from build123d import *

# Parameters (mm, degrees)
SKETCH1_W                  = 60
SKETCH1_H                  = 60
BOSS_EXTRUDE1_DEPTH        = 80
CUT_EXTRUDE2_START         = -16
SKETCH3_R                  = 11
CUT_EXTRUDE2_DEPTH         = 107.553851381
SKETCH4_OUTSIDE_W          = 105.324
SKETCH4_OUTSIDE_H          = 85.324
SKETCH4_OUTSIDE_W_2        = 47.6
SKETCH4_OUTSIDE_H_2        = 47.6
CUT_EXTRUDE5_DEPTH         = 13
M4_TAPPED_HOLE2_AT_2_COUNT = 2
M4_TAPPED_HOLE2_AT_2_PITCH = 20.8
CIRPATTERN2_COUNT          = 4
CIRPATTERN4_COUNT          = 4
SKETCH21_R                 = 8
CUT_EXTRUDE6_DEPTH         = 77.785415282
SKETCH24_W                 = 10
SKETCH24_H                 = 60
CUT_EXTRUDE7_DEPTH         = 53
SKETCH25_W                 = 60
SKETCH25_H                 = 60
BOSS_EXTRUDE2_DEPTH        = 11
FILLET1_R                  = 2


with BuildPart() as part:
    # Sketch1 → Boss-Extrude1 (new body)
    with BuildSketch(Plane.XY):
        Rectangle(SKETCH1_W, SKETCH1_H)
    extrude(amount=BOSS_EXTRUDE1_DEPTH)

    # Sketch3 → Cut-Extrude2 (cut)
    with BuildSketch(Plane(origin=(0, 0, 0), x_dir=(-1, 0, 0), z_dir=(0, 0, -1)).offset(CUT_EXTRUDE2_START)):
        with Locations(Location((-12, 0, 0), (0, 0, 180))):
            Circle(SKETCH3_R)
    cut_extrude2 = extrude(amount=CUT_EXTRUDE2_DEPTH, mode=Mode.SUBTRACT)

    # Sketch4 outside → Cut-Extrude5 (cut)
    with BuildSketch(Plane.ZY.offset(30)):
        with Locations((40, 0)):
            Rectangle(SKETCH4_OUTSIDE_W, SKETCH4_OUTSIDE_H)
        with Locations((40, 0)):
            Rectangle(SKETCH4_OUTSIDE_W_2, SKETCH4_OUTSIDE_H_2, mode=Mode.SUBTRACT)
    extrude(amount=-CUT_EXTRUDE5_DEPTH, mode=Mode.SUBTRACT)

    # Sketch19 → M4 Tapped Hole2 (revolve, cut)
    with BuildSketch(Plane(origin=(-24, -23.8, 29.6), x_dir=(0, 0, -1), z_dir=(1, 0, 0))):
        Polygon((0, 0), (0, 12.491420021), (1.65, 11.5), (1.65, 0), align=None)
    m4_tapped_hole2 = revolve(axis=Axis((-24, -30.15, 29.6), (0, 1, 0)), mode=Mode.SUBTRACT)

    # M4 Tapped Hole2 at 2: M4 Tapped Hole2 ×2
    with Locations(*[(0, 0, i * M4_TAPPED_HOLE2_AT_2_PITCH) for i in range(1, M4_TAPPED_HOLE2_AT_2_COUNT)]):
        add(m4_tapped_hole2, mode=Mode.SUBTRACT)

    # CirPattern2: M4 Tapped Hole2 ×4 about axis
    cirpattern2_axis = Axis((-30, 0, 40), (1, 0, 0))
    for i in range(1, CIRPATTERN2_COUNT):
        add(m4_tapped_hole2.rotate(cirpattern2_axis, i * 360 / CIRPATTERN2_COUNT), mode=Mode.SUBTRACT)

    # CirPattern2 copy 1 sketch → CirPattern2 copy 1 (revolve, cut)
    with BuildSketch(Plane(origin=(-24, -10.4, 16.2), x_dir=(0, 1, 0), z_dir=(1, 0, 0))):
        Polygon((0, 0), (0, 12.491420021), (1.65, 11.5), (1.65, 0), align=None)
    revolve(axis=Axis((-24, -10.4, 9.85), (0, 0, 1)), mode=Mode.SUBTRACT)

    # CirPattern2 copy 2 sketch → CirPattern2 copy 2 (revolve, cut)
    with BuildSketch(Plane(origin=(-24, 23.8, 29.6), x_dir=(0, 0, 1), z_dir=(1, 0, 0))):
        Polygon((0, 0), (0, 12.491420021), (1.65, 11.5), (1.65, 0), align=None)
    revolve(axis=Axis((-24, 30.15, 29.6), (0, -1, 0)), mode=Mode.SUBTRACT)

    # CirPattern2 copy 3 sketch → CirPattern2 copy 3 (revolve, cut)
    with BuildSketch(Plane(origin=(-24, 10.4, 63.8), x_dir=(0, -1, 0), z_dir=(1, 0, 0))):
        Polygon((0, 0), (0, 12.491420021), (1.65, 11.5), (1.65, 0), align=None)
    revolve(axis=Axis((-24, 10.4, 70.15), (0, 0, -1)), mode=Mode.SUBTRACT)

    # Mirror2: Cut-Extrude2 across plane
    add(cut_extrude2.mirror(Plane(origin=(0, 0, 40), x_dir=(1, 0, 0), z_dir=(0, 0, -1))), mode=Mode.SUBTRACT)

    # Sketch23 → M3 Tapped Hole1 (revolve, cut)
    with BuildSketch(Plane.YZ.offset(26.073090354)):
        Polygon((0, 0), (0, 25.751075774), (1.25, 25), (1.25, 0), align=None)
    m3_tapped_hole1 = revolve(axis=Axis((26.073090354, 0, -6.35), (0, 0, 1)), mode=Mode.SUBTRACT)

    # CirPattern4: M3 Tapped Hole1 ×4 about axis
    cirpattern4_axis = Axis((12, 0, 0), (0, 0, 1))
    for i in range(1, CIRPATTERN4_COUNT):
        add(m3_tapped_hole1.rotate(cirpattern4_axis, i * 360 / CIRPATTERN4_COUNT), mode=Mode.SUBTRACT)

    # Mirror3: M3 Tapped Hole1 across plane
    add(m3_tapped_hole1.mirror(Plane(origin=(0, 0, 40), x_dir=(1, 0, 0), z_dir=(0, 0, -1))), mode=Mode.SUBTRACT)

    # Mirror3 copy 1 sketch → Mirror3 copy 1 (revolve, cut)
    with BuildSketch(Plane(origin=(12, 14.073090354, 80), x_dir=(-1, 0, 0), z_dir=(0, 1, 0))):
        Polygon((0, 0), (0, -25.751075774), (1.25, -25), (1.25, 0), align=None)
    revolve(axis=Axis((12, 14.073090354, 86.35), (0, 0, 1)), mode=Mode.SUBTRACT)

    # Mirror3 copy 2 sketch → Mirror3 copy 2 (revolve, cut)
    with BuildSketch(Plane(origin=(-2.073090354, 0, 80), x_dir=(0, -1, 0), z_dir=(-1, 0, 0))):
        Polygon((0, 0), (0, -25.751075774), (1.25, -25), (1.25, 0), align=None)
    revolve(axis=Axis((-2.073090354, 0, 86.35), (0, 0, 1)), mode=Mode.SUBTRACT)

    # Mirror3 copy 3 sketch → Mirror3 copy 3 (revolve, cut)
    with BuildSketch(Plane(origin=(12, -14.073090354, 80), x_dir=(1, 0, 0), z_dir=(0, -1, 0))):
        Polygon((0, 0), (0, -25.751075774), (1.25, -25), (1.25, 0), align=None)
    revolve(axis=Axis((12, -14.073090354, 86.35), (0, 0, 1)), mode=Mode.SUBTRACT)

    # Sketch21 → Cut-Extrude6 (cut, through all)
    with BuildSketch(Plane(origin=(0, 0, 16), x_dir=(-1, 0, 0), z_dir=(0, 0, -1))):
        with Locations((-12, 0)):
            Circle(SKETCH21_R)
    extrude(amount=-CUT_EXTRUDE6_DEPTH, mode=Mode.SUBTRACT)

    # Sketch24 → Cut-Extrude7 (cut)
    with BuildSketch(Plane(origin=(30, 0, 0), x_dir=(0, 0, -1), z_dir=(1, 0, 0))):
        with Locations((-5, 0)):
            Rectangle(SKETCH24_W, SKETCH24_H)
        with Locations((-75, 0)):
            Rectangle(SKETCH24_W, SKETCH24_H)
    extrude(amount=-CUT_EXTRUDE7_DEPTH, mode=Mode.SUBTRACT)

    # Sketch25 → Boss-Extrude2 (add)
    with BuildSketch(Plane(origin=(30, 0, 0), x_dir=(0, 0, -1), z_dir=(1, 0, 0))):
        with Locations((-40, 0)):
            Rectangle(SKETCH25_W, SKETCH25_H)
    extrude(amount=BOSS_EXTRUDE2_DEPTH)

    # Fillet1
    fillet1_edges = [part.edges().sort_by_distance(p)[0] for p in [
        (-17, 30, 40),
        (-17, -30, 40),
        (-17, 0, 10),
        (12, -30, 10),
        (12, 30, 10),
        (-17, 0, 70),
        (12, 30, 70),
        (12, -30, 70),
        (41, 0, 10),
        (41, 30, 40),
        (41, 0, 70),
        (41, -30, 40),
    ]]
    fillet(fillet1_edges, radius=FILLET1_R)


solid = part.part
Model file for the job. Use its own axes, mm. A direction names the side the tool comes from. Coordinates: 2 decimals unless noted, no trailing zeros. Write each loop counter-clockwise with the first axis right and the second up, starting at its lowest first coordinate (ties: lowest second). Pieces come first, ordered by that corner, then holes. Notation, with made-up numbers: (-19, -6.75) - (-4, -6.75) arc R18 cw to (-4, 20.25) - close; hole circle Ø8 at (3, 16). An arc over 180 degrees is marked (long way). Write each question's results on one line, items separated by ' | '. Start each with the question number.
1) 3-axis set-ups, long thin cutter, end or side, ignore diameter. For faces 1 (the face through (-24, -23.8, 40)), 2 (the face through (10, 8, 16)), 3 (the face through (-25.636, 10.615, 58.13)): which of +Z, -Z, +X, -X, +Y, -Y reach the whole face in a straight line?
2) Cut at C-C (x = 5.5). Write the cut outline in (y, z).
3) Cut at A-A (z = 35). Write the cut outline in (x, y), then the cut area to 3 significant figures.
4) Probe line 1 along Y through (x, z) = (-24, 58); line 2 along X through (y, z) = (-10.4, 58); line 3 along Y through (x, z) = (-22, 26.5). List the from-to ranges inside material, lowest first. Write a range as from..to.
5) Flat gauge pins, fed straight in: P1, Ø5, axis at x = -22, y = 23, coming from the +Z side; P2, Ø4, axis at x = -21.5, y = 3.5, coming from the -Z side; P3, Ø3, axis at x = -2.07, y = 0, coming from the -Z side; P4, Ø3, axis at x = -24, z = 29.6, coming from the -Y side. Where does each tip first touch, or does it go through?
6) Cut at D-D (z = 66.5). Write the cut outline in (x, y).
7) Cut at B-B (y = -5.5). Write the cut outline in (x, z), then the cut area to 3 significant figures.
8) Mould opens along Z. For faces 4 (the face through (-25.39, 18.13, 30.49)), 5 (the face through (-24, 0, 63.8)), 6 (the face through (-16.4, -0.39, 10.57)), 7 (the face through (-16.4, -29.43, 40.39)) say: pulls with the +Z half, pulls with the -Z half, needs draft (parallel to the pull), parting line crosses it, or undercut.
Returned:
1) face 1: +Z, -Z, -X, -Y | face 2: -Z | face 3: +Z
2) outline: (-30, 12) arc R2 ccw to (-28, 10) - (-8.87, 10) - (-8.87, 16) - (-4.66, 16) - (-4.66, 64) - (-8.87, 64) - (-8.87, 70) - (-28, 70) arc R2 ccw to (-30, 68) - close; (4.66, 16) - (8.87, 16) - (8.87, 10) - (28, 10) arc R2 ccw to (30, 12) - (30, 68) arc R2 ccw to (28, 70) - (8.87, 70) - (8.87, 64) - (4.66, 64) - close
3) outline: (-30, -23.8) - (-17, -23.8) - (-17, -28) arc R2 ccw to (-15, -30) - (39, -30) arc R2 ccw to (41, -28) - (41, 28) arc R2 ccw to (39, 30) - (-15, 30) arc R2 ccw to (-17, 28) - (-17, 23.8) - (-30, 23.8) - close; hole circle Ø16 at (12, 0) | area: 3,890 mm^2
4) line 1: -23.8..-12.05, -8.75..8.75, 12.05..23.8 | line 2: -30..-25.65, -22.35..41 | line 3: -23.8..23.8
5) P1: z = 63.8 | P2: z = 16.2 | P3: z = 10 | P4: y = -12.21
6) outline: (-17, -28) arc R2 ccw to (-15, -30) - (39, -30) arc R2 ccw to (41, -28) - (41, 28) arc R2 ccw to (39, 30) - (-15, 30) arc R2 ccw to (-17, 28) - close; hole circle Ø2.5 at (-2.07, 0); hole circle Ø22 at (12, 0); hole circle Ø2.5 at (12, -14.07); hole circle Ø2.5 at (12, 14.07); hole circle Ø2.5 at (26.07, 0)
7) outline: (-30, 16.2) - (-17, 16.2) - (-17, 12) arc R2 ccw to (-15, 10) - (2.47, 10) - (2.47, 16) - (6.19, 16) - (6.19, 64) - (2.47, 64) - (2.47, 70) - (-15, 70) arc R2 ccw to (-17, 68) - (-17, 63.8) - (-30, 63.8) - close; (17.81, 16) - (21.53, 16) - (21.53, 10) - (39, 10) arc R2 ccw to (41, 12) - (41, 68) arc R2 ccw to (39, 70) - (21.53, 70) - (21.53, 64) - (17.81, 64) - close | area: 3,310 mm^2
8) face 4: undercut | face 5: pulls with the +Z half | face 6: pulls with the -Z half | face 7: needs draft
